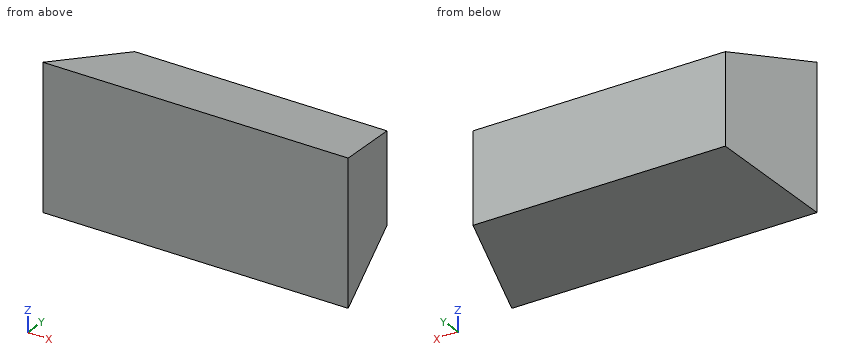
from build123d import *

# Parameters (mm, degrees)
ESQUISSE2_W      = 150
ESQUISSE2_H      = 70
EXTRUSION1_DEPTH = 48.5
EXTRUSION2_REACH = 174.488
CHANFREIN1_SIZE2 = 48.5
CHANFREIN1_SIZE  = 12.995535833
CHANFREIN2_SIZE2 = 48.5
CHANFREIN2_SIZE  = 12.995535833


with BuildPart() as part:
    # Esquisse2 → Extrusion1 (new body)
    with BuildSketch(Plane(origin=(0, 0, 0), x_dir=(1, 0, 0), z_dir=(0, 1, 0))):
        with Locations((75, 35)):
            Rectangle(ESQUISSE2_W, ESQUISSE2_H)
    extrude(amount=EXTRUSION1_DEPTH)

    # Esquisse3 → Extrusion2 (cut, up to next)
    with BuildSketch(Plane.XY, mode=Mode.PRIVATE) as extrusion2_sk1:
        Polygon((0, 0), (0, 48.5), (12.995535833, 48.5), align=None)
    extrusion2_tool1 = extrude(extrusion2_sk1.sketch, amount=-EXTRUSION2_REACH, mode=Mode.PRIVATE) & part.part
    # Esquisse3 → Extrusion2 (cut, up to next)
    with BuildSketch(Plane.XY, mode=Mode.PRIVATE) as extrusion2_sk2:
        Polygon((137.004464167, 48.5), (150, 0), (150, 48.5), align=None)
    extrusion2_tool2 = extrude(extrusion2_sk2.sketch, amount=-EXTRUSION2_REACH, mode=Mode.PRIVATE) & part.part
    add(extrusion2_tool1.solids().sort_by_distance((4.331845, 32.333333, 0))[0], mode=Mode.SUBTRACT)
    add(extrusion2_tool2.solids().sort_by_distance((145.668155, 32.333333, 0))[0], mode=Mode.SUBTRACT)

    # Chanfrein1
    chanfrein1_edges = [part.edges().sort_by_distance(p)[0] for p in [
        (75, 48.5, -70),
    ]]
    chanfrein1_side = [part.faces().sort_by_distance(p)[0] for p in [
        (75, 48.5, -69.740089283),
    ]]
    chamfer(chanfrein1_edges, length=CHANFREIN1_SIZE - 0.0001, length2=CHANFREIN1_SIZE2 - 0.0001, reference=chanfrein1_side[0])  # a hair under: the kernel refuses the full size

    # Chanfrein2
    chanfrein2_edges = [part.edges().sort_by_distance(p)[0] for p in [
        (75, 48.5, 0),
    ]]
    chanfrein2_side = [part.faces().sort_by_distance(p)[0] for p in [
        (75, 48.5, -0.259910717),
    ]]
    chamfer(chanfrein2_edges, length=CHANFREIN2_SIZE - 0.0001, length2=CHANFREIN2_SIZE2 - 0.0001, reference=chanfrein2_side[0])  # a hair under: the kernel refuses the full size


solid = part.part
The listing builds one solid part. Answer for the finished solid, in the listing's coordinates (mm). Coordinates: 2 decimals unless noted, no trailing zeros. Loops run counter-clockwise (first coordinate to the right, second up) from the corner with the lowest first, then second, coordinate; pieces in that order, holes last.
1) Find section C-C on y = 23. Write down the section's boundary in (x, z), then the cut area to 3 significant figures.
2) Find the intervals of material crossed by L1, parallel to Z at x = 17, y = 37; L2, parallel to Z at x = 33.5, y = 29.5; L3, parallel to X at y = 15, z = -39, in increasing order.
3) Find section A-A on z = -37. Write down the section's boundary in (x, y).
4) Flat-ended cylindrical pins translate along their axes: pin 1 Ø5 at (x, z) = (96, -59) entering from +Y; pin 2 Ø4 at (x, y) = (67, 22.5) entering from +Z; pin 3 Ø1.5 at (y, z) = (6.5, -59.5) entering from +X; pin 4 Ø1 at (y, z) = (42, -49) entering from -X. Find the tip coordinate at first contact, or state that the pin passes through.
Values:
1. outline: (6.16, -63.84) - (143.84, -63.84) - (143.84, -6.16) - (6.16, -6.16) - close
1. area: 7,940 mm2
2. L1: z = -60.09 to -9.91
2. L2: z = -62.1 to -7.9
2. L3: x = 4.02 to 145.98
3. outline: (0, 0) - (150, 0) - (137, 48.5) - (13, 48.5) - close
4. pin 1: stops at y = 48.5
4. pin 2: stops at z = -5.49
4. pin 3: stops at x = 148.46
4. pin 4: stops at x = 11.12
